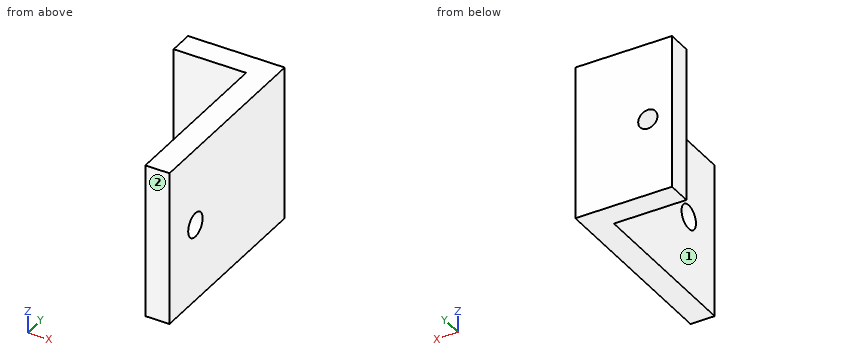
```python
from build123d import *

# Parameters (mm, degrees)
BOSS_EXTRUDE1_DEPTH         = 40.64
F_1_4_0_25_DIAMETER_HOLE1_D = 6.35
F_8_0_199_DIAMETER_HOLE2_D  = 5.0546


with BuildPart() as part:
    # Sketch1 → Boss-Extrude1 (new body)
    with BuildSketch(Plane.XY):
        Polygon((-17.365909091, 21.527272727), (8.034090909, 21.527272727), (8.034090909, 12.565909091), (8.034090909, -29.272727273), (1.684090909, -29.272727273), (1.684090909, 15.177272727), (-17.365909091, 15.177272727), align=None)
    extrude(amount=BOSS_EXTRUDE1_DEPTH)

    # 1/4 (0.25) Diameter Hole1 (through all)
    with Locations(Plane(origin=(8.034090909, 0, 0), x_dir=(0, 0, -1), z_dir=(1, 0, 0))):
        with Locations((-20.32, -17.842727273)):
            Hole(F_1_4_0_25_DIAMETER_HOLE1_D / 2)

    # #8 (0.199) Diameter Hole2 (through all)
    with Locations(Plane(origin=(0, 21.527272727, 0), x_dir=(1, 0, 0), z_dir=(0, 1, 0))):
        with Locations((-11.015909091, -20.32)):
            Hole(F_8_0_199_DIAMETER_HOLE2_D / 2)


solid = part.part
```
Source: CAD feature listing. Evaluate the final solid. Frame: model axes, mm. Face numbers are marked on the shaded views. A direction names the side the tool comes from. Round coordinates to 2 decimals unless told otherwise and drop trailing zeros. Loops run counter-clockwise (first coordinate to the right, second up) from the corner with the lowest first, then second, coordinate; pieces in that order, holes last. Notation, with made-up numbers: M 32,46 L 67,46 A18 cw 67,54 Z; hole C 45.5,-28.5 d9. An arc over 180 degrees is marked long. Use a Markdown table: item, result. Add a question column.
1. Reachability of the marked faces 1 and 2 from +Z, -Z, +X, -X, +Y, -Y: full face, straight path, thin tool, end or side. Return the list, or none.
2. Section query A-A on z = 20.32. Return the cut outline in (x, y), then the cut area to 3 significant figures.
3. Section query B-B on y = 18. Return the cut outline in (x, z).
4. Line query: line 1 (Y direction, x = 6, z = 20.32); line 2 (X direction, y = 17.5, z = 20.32); line 3 (Y direction, x = -3.5, z = 8.5). Output: solid intervals per line, ascending.
5. Section query D-D on z = 14. Return the cut outline in (x, y).
6. Contact query for a flat-ended pin moving along its axis: P1, Ø15, axis at x = -7.5, z = 13, coming from the -Y side. Output: stop coordinate, or through.
7. Section query C-C on x = -10.25. Return the cut outline in (y, z), then the cut area to 3 significant figures.
Reported:
| question | item | result |
|---|---|---|
| 1 | face 1 | +Z, -Z, -X, -Y |
| 1 | face 2 | +Z, -Z, +X, -X, -Y |
| 2 | outline | M -17.37,15.18 L -13.54,15.18 L -13.54,21.53 L -17.37,21.53 Z; M -8.49,15.18 L 1.68,15.18 L 1.68,-14.67 L 8.03,-14.67 L 8.03,21.53 L -8.49,21.53 Z; M 1.68,-29.27 L 8.03,-29.27 L 8.03,-21.02 L 1.68,-21.02 Z |
| 2 | area | 371 mm² |
| 3 | outline | M -17.37,0 L 8.03,0 L 8.03,40.64 L -17.37,40.64 Z; hole C -11.02,20.32 d5.05 |
| 4 | line 1 | y = -29.27 to -21.02, -14.67 to 21.53 |
| 4 | line 2 | x = -17.37 to -13.54, -8.49 to 8.03 |
| 4 | line 3 | y = 15.18 to 21.53 |
| 5 | outline | M -17.37,15.18 L 1.68,15.18 L 1.68,-29.27 L 8.03,-29.27 L 8.03,21.53 L -17.37,21.53 Z |
| 6 | P1 | stops at y = 15.18 |
| 7 | outline | M 15.18,0 L 21.53,0 L 21.53,17.91 L 15.18,17.91 Z; M 15.18,22.73 L 21.53,22.73 L 21.53,40.64 L 15.18,40.64 Z |
| 7 | area | 227 mm² |
